from build123d import *

# Parameters (mm, degrees)
SKETCH_1_W          = 46
SKETCH_1_H          = 31.5
EXTRUDE_1_DEPTH     = 18
SKETCH_3_W          = 3.3
SKETCH_3_H          = 13
EXTRUDE_2_DEPTH     = 8.5
SKETCH_4_W          = 3.3
SKETCH_4_H          = 13
EXTRUDE_3_DEPTH     = 8.5
CUT_EXTRUDE_1_DEPTH = 65.642014201
CUT_EXTRUDE_2_DEPTH = 65.642014201


with BuildPart() as part:
    # 草图1 → 凸台-拉伸1 (new body)
    with BuildSketch(Plane.XY):
        with Locations((23, 15.75)):
            Rectangle(SKETCH_1_W, SKETCH_1_H)
    extrude(amount=EXTRUDE_1_DEPTH)

    # 草图3 → 凸台-拉伸2 (add)
    with BuildSketch(Plane.ZY):
        with Locations((1.65, 15.75)):
            Rectangle(SKETCH_3_W, SKETCH_3_H)
    extrude(amount=EXTRUDE_2_DEPTH)

    # 草图4 → 凸台-拉伸3 (add)
    with BuildSketch(Plane(origin=(46, 0, 0), x_dir=(0, 0, -1), z_dir=(1, 0, 0))):
        with Locations((-1.65, 15.75)):
            Rectangle(SKETCH_4_W, SKETCH_4_H)
    extrude(amount=EXTRUDE_3_DEPTH)

    # 草图5 → 切除-拉伸1 (cut, through all)
    with BuildSketch(Plane.XY.offset(3.3)):
        Polygon((-8.5, 22.25), (-8.5, 20), (0, 22.25), align=None)
        Polygon((-8.5, 11.5), (0, 9.25), (-8.5, 9.25), align=None)
        with BuildLine():
            Line((-3, 17.75), (-8.5, 17.75))
            Line((-8.5, 17.75), (-8.5, 13.75))
            Line((-8.5, 13.75), (-3, 13.75))
            ThreePointArc((-3, 13.75), (-1, 15.75), (-3, 17.75))
        make_face()
    extrude(amount=-CUT_EXTRUDE_1_DEPTH, mode=Mode.SUBTRACT)

    # 草图6 → 切除-拉伸2 (cut, through all)
    with BuildSketch(Plane.XY.offset(3.3)):
        Polygon((46, 22.25), (54.5, 20), (54.5, 22.25), align=None)
        Polygon((46, 9.25), (54.5, 9.25), (54.5, 11.5), align=None)
        with BuildLine():
            Line((49, 17.75), (54.5, 17.75))
            Line((54.5, 17.75), (54.5, 13.75))
            Line((54.5, 13.75), (49, 13.75))
            ThreePointArc((49, 13.75), (47, 15.75), (49, 17.75))
        make_face()
    extrude(amount=-CUT_EXTRUDE_2_DEPTH, mode=Mode.SUBTRACT)


solid = part.part
The listing builds one solid part. Answer for the finished solid, in the listing's coordinates (mm). A direction names the side the tool comes from. Give positions to 0.01 mm unless a question says otherwise; leave off trailing zeros. Loops run counter-clockwise (first coordinate to the right, second up) from the corner with the lowest first, then second, coordinate; pieces in that order, holes last. Notation, with made-up numbers: (75, 58) - (104, 58) arc R21 cw to (104, 68) - close; hole circle Ø4 at (81.5, 48.25). An arc over 180 degrees is marked (long way). Answer as a JSON object with one key per item and string values.
1. A cutting plane is placed at C-C (y = 10.5). Write down the section's boundary in (x, z).
Determined:
{"outline": "(-4.72, 0) - (50.72, 0) - (50.72, 3.3) - (46, 3.3) - (46, 18) - (0, 18) - (0, 3.3) - (-4.72, 3.3) - close"}
2. Flat-ended cylindrical pins translate along their axes: pin 1 Ø1.5 at (x, y) = (-2, 20) entering from -Z; pin 2 Ø2.5 at (x, y) = (-3.5, 15.5) entering from +Z; pin 3 Ø2.5 at (x, y) = (52, 13) entering from +Z; pin 4 Ø2 at (y, z) = (5, 8) entering from +X. Find the tip coordinate at first contact, or state that the pin passes through.
Determined:
{"pin 1": "z = 0", "pin 2": "through", "pin 3": "z = 3.3", "pin 4": "x = 46"}
3. For faces 1 (the flat face through (-1, 17, 3.3)), 2 (the flat face through (-6, 13.75, 2)), 3 (the flat face through (52, 17.75, 2)), determine the directions among +Z, -Z, +X, -X, +Y, -Y from which every point of the face is accessible in a straight line to the end or side of a thin tool.
Determined:
{"face 1": "+Z, -X, +Y, -Y", "face 2": "+Z, -Z, -X", "face 3": "+Z, -Z, +X"}
4. Find the intervals of material crossed by L1, parallel to X at y = 9, z = 8.75; L2, parallel to Z at x = -2, y = 12, in increasing order. Write a range as [from, to].
Determined:
{"L1": "[0, 46]", "L2": "[0, 3.3]"}
5. A cutting plane is placed at B-B (z = 16.5). Write down the section's boundary in (x, y).
Determined:
{"outline": "(0, 0) - (46, 0) - (46, 31.5) - (0, 31.5) - close"}
6. For a pull along Y with two mould halves and no side action, classify faces 4 (the flat face through (-6, 17.75, 2)), 5 (the flat face through (23, 0, 9)), 6 (the flat face through (47, 17, 3.3)), 7 (the flat face through (50.19, 21.14, 1.67)) as pulls with the +Y half, pulls with the -Y half, needs draft (parallel to the pull), parting line crosses it, or undercut.
Determined:
{"face 4": "undercut", "face 5": "pulls with the -Y half", "face 6": "needs draft", "face 7": "pulls with the +Y half"}
7. A cutting plane is placed at A-A (y = 15.75). Write down the section's boundary in (x, z), then the cut area to 3 significant figures.
Determined:
{"outline": "(-1, 0) - (47, 0) - (47, 3.3) - (46, 3.3) - (46, 18) - (0, 18) - (0, 3.3) - (-1, 3.3) - close", "area": "835 mm²"}
8. A cutting plane is placed at D-D (y = 7). Write down the section's boundary in (x, z), then the cut area to 3 significant figures.
Determined:
{"outline": "(0, 0) - (46, 0) - (46, 18) - (0, 18) - close", "area": "828 mm²"}
